The listing builds one solid part. Answer for the finished solid, in the listing's coordinates (mm). Face numbers are marked on the shaded views. A direction names the side the tool comes from. Coordinates: 2 decimals unless noted, no trailing zeros. Order: outer loops, then holes, each group sorted by start corner. A loop starts at its lowest first (then second) coordinate and runs counter-clockwise, first axis right, second up. Notation, with made-up numbers: (-36, -39.5) - (-17, -39.5) arc R19 cw to (-17, -29.5) - close; hole circle Ø2 at (-17, 49). An arc over 180 degrees is marked (long way). Use a Markdown table: item, result. Add a question column.
Item 1: Flat-ended cylindrical pins translate along their axes: P1, Ø7.5, axis at x = -15, y = -12.5, coming from the +Z side; P2, Ø5, axis at x = -9.5, y = 3, coming from the -Z side; P3, Ø2, axis at y = -3, z = 2.5, coming from the -X side. Find the tip coordinate at first contact, or state that the pin passes through.
Item 2: For the marked faces 5 and 6, determine the directions among +Z, -Z, +X, -X, +Y, -Y from which every point of the face is accessible in a straight line to the end or side of a thin tool.
Item 3: The mould has two halves that part along Y. Classify the marked faces 1, 2, 3 and 4: released by +Y, released by -Y, zero draft, split by the parting line, or undercut.
Item 4: The part is cut by section B-B, the plane y = -18. Give the vertices of the cut face in (x, z).
Item 5: The part is cut by section A-A, the plane z = 8.5. State how many separate pieces and enclosed holes the cut face has, then the cut area to 3 significant figures.
Item 6: Find the intervals of material crossed by line 1 along X through (y, z) = (-24, 12.25); line 2 along Z through (x, y) = (-21.75, 1); line 3 along X through (y, z) = (-11, 6), in increasing order.
from build123d import *

# Parameters (mm, degrees)
F0_W     = 25
F0_H     = 34.8
F1_DEPTH = 12.5
F3_START = -2.2
F2_R     = 10.35
F3_DEPTH = 30.4
F4_W     = 20.7
F4_H     = 1.52
F5_DEPTH = 10.6
F6_R     = 5
F7_R     = 2
F9_DEPTH = 2


with BuildPart() as f1:
    # F0 (on Top) → F1 (new body)
    with BuildSketch(Plane.XY):
        with Locations((-17.5982150249, -9.7193448131)):
            Rectangle(F0_W, F0_H)
    extrude(amount=F1_DEPTH)

    # F2 (on face) → F3 (cut)
    with BuildSketch(Plane.XZ.offset(27.1193448131).offset(F3_START)):
        with Locations((-17.5982150249, 12.5)):
            Circle(F2_R)
    extrude(amount=-F3_DEPTH, mode=Mode.SUBTRACT)

    # F4 (on face) → F5 (join)
    with BuildSketch(Plane.XY.offset(12.5)):
        with Locations((-17.5982150249, 0.9206551869)):
            Rectangle(F4_W, F4_H)
        with Locations((-17.5982150249, -4.3993448131)):
            Rectangle(F4_W, F4_H)
        with Locations((-17.5982150249, -9.7193448131)):
            Rectangle(F4_W, F4_H)
        with Locations((-17.5982150249, -15.0393448131)):
            Rectangle(F4_W, F4_H)
        with Locations((-17.5982150249, -20.3593448131)):
            Rectangle(F4_W, F4_H)
    extrude(amount=-F5_DEPTH)

    # F6
    f6_edges = [f1.edges().sort_by_distance(p)[0] for p in [
        (-5.098215, -9.719345, 0),
        (-30.098215, -9.719345, 0),
    ]]
    fillet(f6_edges, radius=F6_R)

    # F7
    f7_edges = [f1.edges().sort_by_distance(p)[0] for p in [
        (-5.098215, -27.119345, 8.75),
        (-5.098215, 7.680655, 8.75),
    ]]
    fillet(f7_edges, radius=F7_R)

    # F8 (on face) → F9 (join)
    with BuildSketch(Plane.XY.offset(12.5)):
        with BuildLine():
            Line((-30.0982150249, 2.1706551869), (-30.0982150249, -0.3293448131))
            ThreePointArc((-30.0982150249, -0.3293448131), (-28.8482150249, 0.9206551869), (-30.0982150249, 2.1706551869))
        make_face()
        with BuildLine():
            Line((-5.0982150249, -0.3293448131), (-5.0982150249, 2.1706551869))
            ThreePointArc((-5.0982150249, 2.1706551869), (-6.3482150249, 0.9206551869), (-5.0982150249, -0.3293448131))
        make_face()
        with BuildLine():
            ThreePointArc((-5.0982150249, -19.1093448131), (-6.3482150249, -20.3593448131), (-5.0982150249, -21.6093448131))
            Line((-5.0982150249, -21.6093448131), (-5.0982150249, -19.1093448131))
        make_face()
        with BuildLine():
            ThreePointArc((-30.0982150249, -21.6093448131), (-28.8482150249, -20.3593448131), (-30.0982150249, -19.1093448131))
            Line((-30.0982150249, -19.1093448131), (-30.0982150249, -21.6093448131))
        make_face()
    extrude(amount=F9_DEPTH)


solid = f1.part
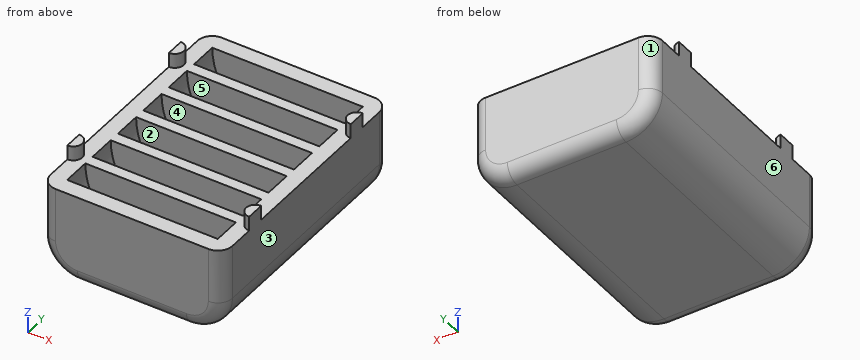
Solution:
| question | item | result |
|---|---|---|
| 1 | P1 | stops at z = 12.5 |
| 1 | P2 | stops at z = 0 |
| 1 | P3 | stops at x = -29.87 |
| 2 | face 5 | +Z |
| 2 | face 6 | +Z, -Z, -X, +Y, -Y |
| 3 | face 1 | released by +Y |
| 3 | face 2 | undercut |
| 3 | face 3 | zero draft |
| 3 | face 4 | undercut |
| 4 | outline | (-30.1, 5) arc R5 ccw to (-25.1, 0) - (-10.1, 0) arc R5 ccw to (-5.1, 5) - (-5.1, 12.5) - (-7.25, 12.5) arc R10.35 cw to (-27.95, 12.5) - (-30.1, 12.5) - close |
| 5 | separate pieces | 1 |
| 5 | enclosed holes | 6 |
| 5 | area | 431 mm2 |
| 6 | line 1 | x = -30.1 to -27.95, -7.25 to -5.1 |
| 6 | line 2 | z = 0 to 12.5 |
| 6 | line 3 | x = -30.1 to -25.65, -9.54 to -5.1 |
